```python
from build123d import *

# Parameters (mm, degrees)
SKETCH1_R                = 11
SKETCH1_R_2              = 3.95
BOSS_EXTRUDE1_DEPTH      = 3.5
BOSS_EXTRUDE1_DEPTH_BACK = 3.5
CUT_EXTRUDE1_START       = -3.5
SKETCH2_R                = 9.75
SKETCH2_R_2              = 5.2
CUT_EXTRUDE1_DEPTH       = 0.25
CUT_EXTRUDE2_START       = 3.5
SKETCH2_2_R              = 9.75
SKETCH2_2_R_2            = 5.2
CUT_EXTRUDE2_DEPTH       = 0.25
CHAMFER1_SIZE            = 0.1


with BuildPart() as part:
    # Sketch1 → Boss-Extrude1 (new body, two sides)
    with BuildSketch(Plane.XY) as boss_extrude1_sk:
        Circle(SKETCH1_R)
        Circle(SKETCH1_R_2, mode=Mode.SUBTRACT)
    extrude(amount=BOSS_EXTRUDE1_DEPTH)
    extrude(boss_extrude1_sk.sketch, amount=-BOSS_EXTRUDE1_DEPTH_BACK)

    # Sketch2 → Cut-Extrude1 (cut)
    with BuildSketch(Plane.XY.offset(CUT_EXTRUDE1_START)):
        Circle(SKETCH2_R)
        Circle(SKETCH2_R_2, mode=Mode.SUBTRACT)
    extrude(amount=CUT_EXTRUDE1_DEPTH, mode=Mode.SUBTRACT)

    # Sketch2<2> → Cut-Extrude2 (cut)
    with BuildSketch(Plane.XY.offset(CUT_EXTRUDE2_START)):
        Circle(SKETCH2_2_R)
        Circle(SKETCH2_2_R_2, mode=Mode.SUBTRACT)
    extrude(amount=-CUT_EXTRUDE2_DEPTH, mode=Mode.SUBTRACT)

    # Chamfer1
    chamfer1_edges = [part.edges().sort_by_distance(p)[0] for p in [
        (-5.2, 0, -3.5),
        (-9.75, 0, -3.5),
        (-9.75, 0, 3.5),
        (-5.2, 0, 3.5),
        (-11, 0, -3.5),
        (-3.95, 0, -3.5),
        (-11, 0, 3.5),
        (-3.95, 0, 3.5),
    ]]
    chamfer(chamfer1_edges, length=CHAMFER1_SIZE)


solid = part.part
```
Could you check a few things on this model? Use its own coordinates, in mm. A direction names the side the tool comes from. Give positions to 0.01 mm unless a question says otherwise; leave off trailing zeros. Order: outer loops, then holes, each group sorted by start corner. A loop starts at its lowest first (then second) coordinate and runs counter-clockwise, first axis right, second up.
Q1. I'm going to push flat-ended pins straight in: P1, Ø7, axis at x = 0, y = 0, coming from the +Z side; P2, Ø1.5, axis at x = 6, z = -1, coming from the +Y side; P3, Ø1.5, axis at x = -8, z = 0, coming from the -Y side; P4, Ø1.5, axis at x = 5.5, y = -3.5, coming from the +Z side. Where does each tip first touch, or does it pass through?
Q2. If I drill on line 1 along Y through (x, z) = (0, -3.3); line 2 along Z through (x, y) = (6.75, -4.75); line 3 along Y through (x, z) = (1.25, -1), over which ranges is the centre line in solid material (lowest first)?
Q3. We'd pull the mould along Y, two halves only. Please class faces 1 (the flat face through (-8, -6, 3.5)), 2 (the flat face through (4, -4, 3.25)): +Y half, -Y half, draft (parallel to the pull), parting line (faces both ways), or undercut.
Q4. For faces 3 (the flat face through (-8, -6, -3.5)), 4 (the flat face through (4, -4, -3.25)), which set-ups out of +Z, -Z, +X, -X, +Y, -Y let a thin tool reach every point of the face, with its end or its side?
Q5. Suppose I cut it at A-A, the plane z = -2.5. Write out the boundary of the cut face in (x, y).
Solution:
1. P1: passes through
1. P2: stops at y = 9.67
1. P3: stops at y = -8.27
1. P4: stops at z = 3.25
2. line 1: y = -11 to -9.75, -5.2 to -3.95, 3.95 to 5.2, 9.75 to 11
2. line 2: z = -3.25 to 3.25
2. line 3: y = -10.93 to -3.75, 3.75 to 10.93
3. face 1: draft
3. face 2: undercut
4. face 3: -Z, +X, -X, +Y, -Y
4. face 4: -Z
5. outline: circle Ø22 at (0, 0); hole circle Ø7.9 at (0, 0)
